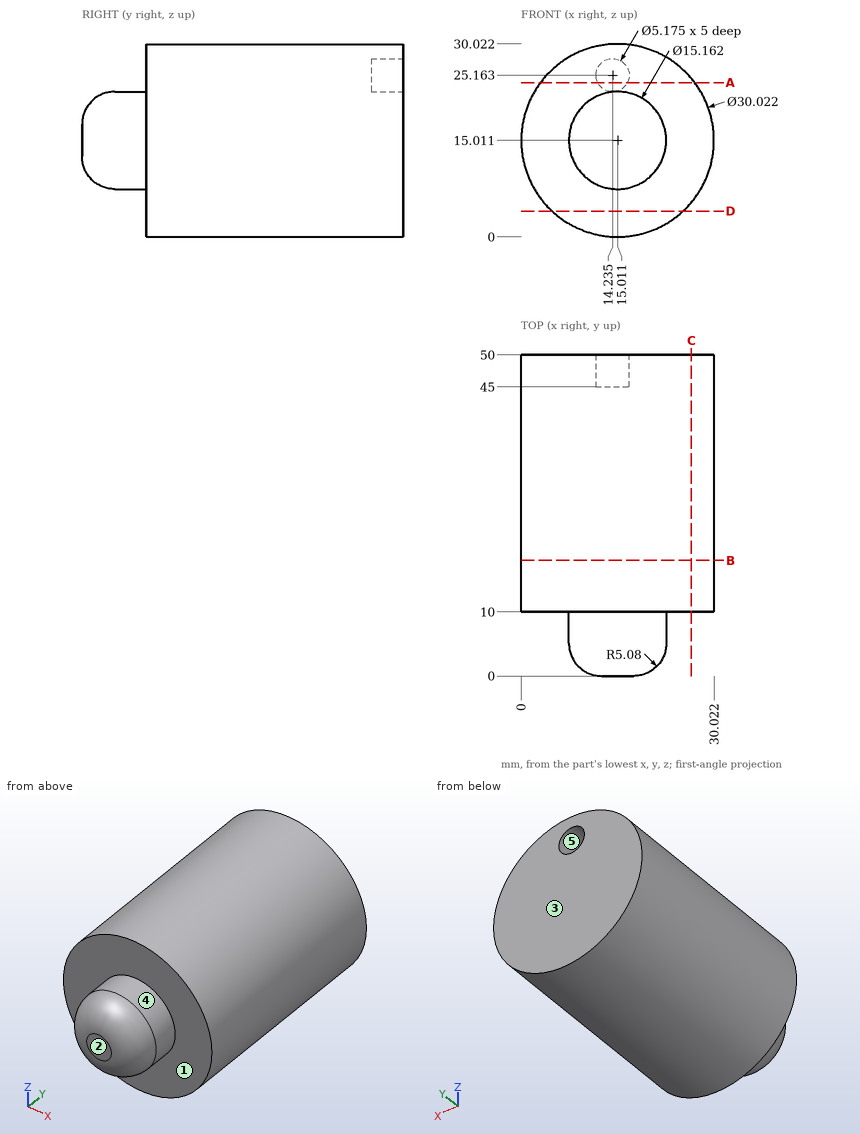
Drawing for the job (mm, zero at the part's lowest x, y, z). A direction names the side the tool comes from. Give positions to 0.01 mm unless a question says otherwise; leave off trailing zeros. Order: outer loops, then holes, each group sorted by start corner. A loop starts at its lowest first (then second) coordinate and runs counter-clockwise, first axis right, second up. Notation, with made-up numbers: M -23,18 L 19,18 A29 ccw 19,54 Z; hole C 6,11.5 d5. An arc over 180 degrees is marked long. Put each result on its own line as item: value. Start each with the question number.
(1) Saw through at B-B, the plane y = 18. Write the cut outline in (x, z).
(2) Flat gauge pins, fed straight in: pin 1 Ø1 at (x, y) = (13.5, 29) entering from -Z; pin 2 Ø4 at (y, z) = (11, 8) entering from +X; pin 3 Ø8 at (y, z) = (35.5, 10) entering from -X. Where does each tip first touch, or does it go through?
(3) Mould opens along Z. For the marked faces 3, 4 and 5 say: +Z half, -Z half, draft (parallel to the pull), parting line (faces both ways), or undercut.
(4) Which spindle directions (+Z, -Z, +X, -X, +Y, -Y) get a long thin tool onto all of the face, cutting with end or side? Do the marked faces 1 and 2. Say none if no direction does.
(5) Saw through at D-D, the plane z = 4. Write the cut outline in (x, y), then the cut area to 3 significant figures.
(6) Saw through at C-C, the plane x = 26.5. Write the cut outline in (y, z).
(7) Saw through at A-A, the plane z = 24. Write the cut outline in (x, y), then the cut area to 3 significant figures.
(8) Drill centre lines: line 1 along Y through (x, z) = (9, 26); line 2 along Z through (x, y) = (15, 22.5); line 3 along Z through (x, y) = (17, 2). Where is each one in solid material? Low to high.
Check result:
1. outline: C 15.01,15.01 d30.02
2. pin 1: stops at z = 0.03
2. pin 2: stops at x = 29.16
2. pin 3: stops at x = 0.03
3. face 3: draft
3. face 4: parting line
3. face 5: undercut
4. face 1: -Y
4. face 2: +Z, -Z, +X, -X, -Y
5. outline: M 4.81,10 L 25.21,10 L 25.21,50 L 4.81,50 Z
5. area: 816 mm2
6. outline: M 10,5.35 L 50,5.35 L 50,24.67 L 10,24.67 Z
7. outline: M 2.99,10 L 27.03,10 L 27.03,50 L 16.55,50 L 16.55,45 L 11.92,45 L 11.92,50 L 2.99,50 Z
7. area: 939 mm2
8. line 1: y = 10 to 50
8. line 2: z = 0 to 30.02
8. line 3: z = 8.78 to 21.24
